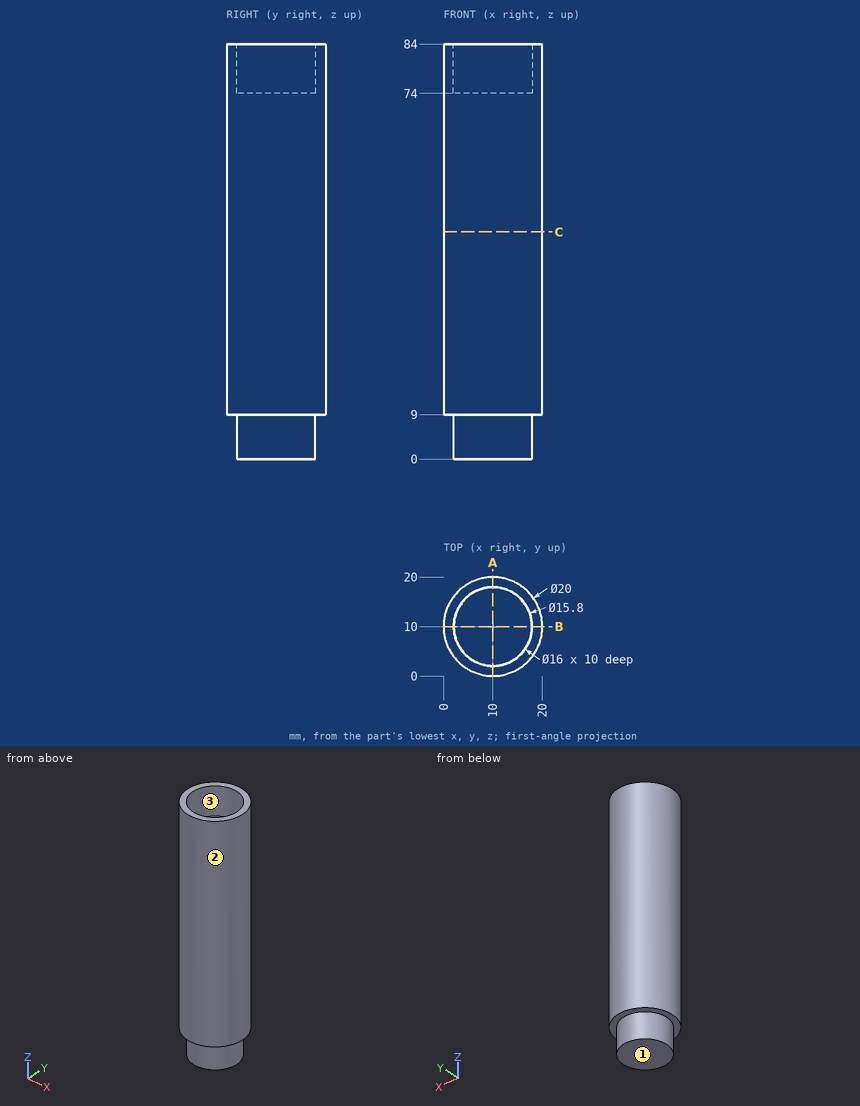
Design review of the part shown in the three views and the two pictorial views. Dimensions are in mm from the part's minimum x, y and z. Coordinates: 2 decimals unless noted, no trailing zeros. Order: outer loops, then holes, each group sorted by start corner. A loop starts at its lowest first (then second) coordinate and runs counter-clockwise, first axis right, second up.
Item 1: For line 1 (Y direction, x = 10, z = 79.75); line 2 (Z direction, x = 13.5, y = 15.75); line 3 (Z direction, x = 8.5, y = 18), list the stretches that pass through material, from the lowest coordinate up.
Item 2: The part is to be moulded in two halves that separate along X. For the marked faces 1, 2 and 3, say which applies: pulls with the +X half, pulls with the -X half, needs draft (parallel to the pull), parting line crosses it, or undercut.
Item 3: Take a section at C-C, the plane z = 46. Write out the cut boundary in (x, y).
Item 4: For pin 1 Ø1 at (y, z) = (9.5, 65.5) entering from -X; pin 2 Ø2 at (x, z) = (4.5, 12.5) entering from +Y, all flat-tipped, find the tip position at first contact; note any pin that passes through.
Item 5: Take a section at A-A, the plane x = 10. Write out the cut boundary in (y, z).
The answers:
1. line 1: y = 0 to 2, 18 to 20
1. line 2: z = 0 to 74
1. line 3: z = 9 to 84
2. face 1: needs draft
2. face 2: parting line crosses it
2. face 3: undercut
3. outline: circle Ø20 at (10, 10)
4. pin 1: stops at x = 0
4. pin 2: stops at y = 18.93
5. outline: (0, 9) - (2.1, 9) - (2.1, 0) - (17.9, 0) - (17.9, 9) - (20, 9) - (20, 84) - (18, 84) - (18, 74) - (2, 74) - (2, 84) - (0, 84) - close
